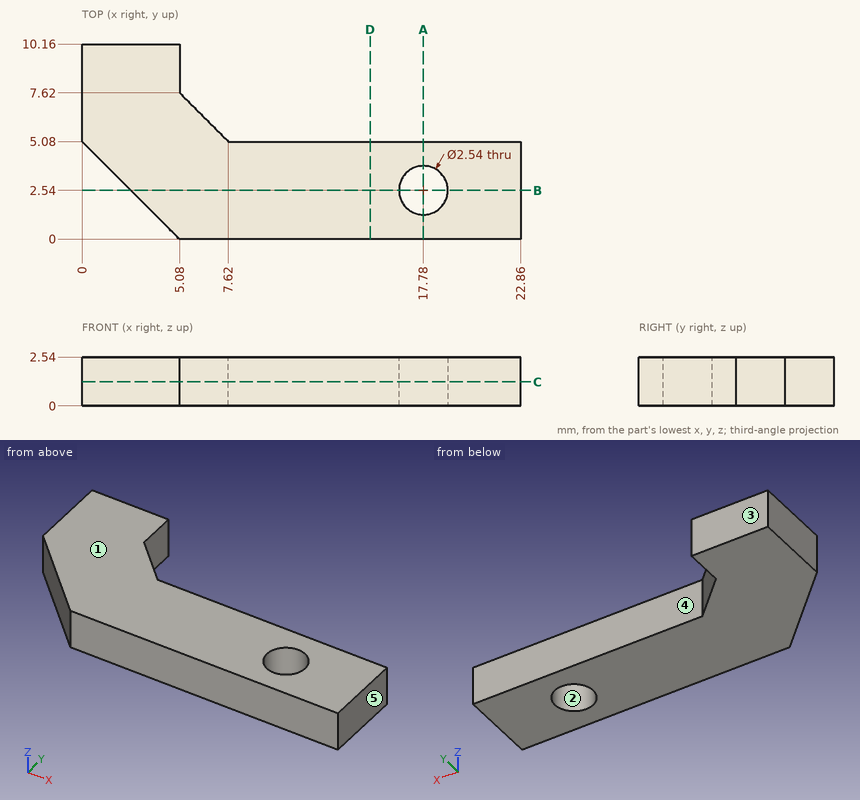
Source: three-view drawing plus pictorial views. Frame: mm from the lowest corner of the part. A direction names the side the tool comes from. Round coordinates to 2 decimals unless told otherwise and drop trailing zeros. Order: outer loops, then holes, each group sorted by start corner. A loop starts at its lowest first (then second) coordinate and runs counter-clockwise, first axis right, second up. Notation, with made-up numbers: (46, 52) -> (67, 52) arc R20 cw to (67, 83) -> close; hole circle Ø3 at (23.25, 14). An arc over 180 degrees is marked (long way). Use one line per item in the form item = value. Start each with the question number.
1. Line query: probe 1 along Y at (x, z) = (17.78, 1.45); probe 2 along X at (y, z) = (8.5, 1.85). Output: solid intervals per line, ascending.
2. Cut plane D-D (x = 15). Return the cut outline in (y, z).
3. Cut plane B-B (y = 2.54). Return the cut outline in (x, z), then the cut area to 3 significant figures.
4. Pin query (flat end, axial travel): pin 1 Ø2 at (x, y) = (9.5, 1) entering from -Z; pin 2 Ø0.8 at (y, z) = (8.5, 1.5) entering from +X; pin 3 Ø0.8 at (x, z) = (12.5, 1) entering from +Y. Return the tip coordinate at first contact, or that it passes through.
5. Draft query along Y for the marked faces 1, 2 and 3. Return one class per face: pulls with the +Y half, pulls with the -Y half, needs draft (parallel to the pull), parting line crosses it, or undercut.
6. Cut plane C-C (z = 1.25). Return the cut outline in (x, y).
7. Cut plane A-A (x = 17.78). Return the cut outline in (y, z), then the cut area to 3 significant figures.
8. Reachability of the marked faces 4 and 5 from +Z, -Z, +X, -X, +Y, -Y: full face, straight path, thin tool, end or side. Return the list, or none.
Solution:
q1.probe_1 = 0 to 1.27, 3.81 to 5.08
q1.probe_2 = 0 to 5.08
q2.outline = (0, 0) -> (5.08, 0) -> (5.08, 2.54) -> (0, 2.54) -> close
q3.outline = (2.54, 0) -> (16.51, 0) -> (16.51, 2.54) -> (2.54, 2.54) -> close; (19.05, 0) -> (22.86, 0) -> (22.86, 2.54) -> (19.05, 2.54) -> close
q3.area = 45.2 mm^2
q4.pin_1 = 0
q4.pin_2 = 5.08
q4.pin_3 = 5.08
q5.face_1 = needs draft
q5.face_2 = undercut
q5.face_3 = pulls with the +Y half
q6.outline = (0, 5.08) -> (5.08, 0) -> (22.86, 0) -> (22.86, 5.08) -> (7.62, 5.08) -> (5.08, 7.62) -> (5.08, 10.16) -> (0, 10.16) -> close; hole circle Ø2.54 at (17.78, 2.54)
q7.outline = (0, 0) -> (1.27, 0) -> (1.27, 2.54) -> (0, 2.54) -> close; (3.81, 0) -> (5.08, 0) -> (5.08, 2.54) -> (3.81, 2.54) -> close
q7.area = 6.45 mm^2
q8.face_4 = +Z, -Z, +X, +Y
q8.face_5 = +Z, -Z, +X, +Y, -Y
